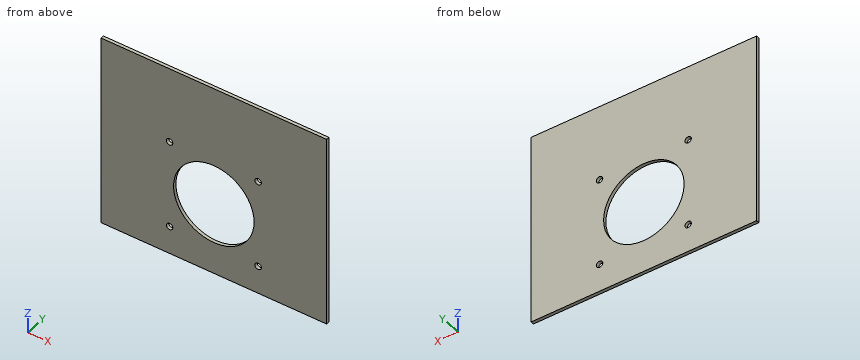
from build123d import *

# Parameters (mm, degrees)
SKETCH_1_W      = 140
SKETCH_1_H      = 120
SKETCH_1_R      = 2
SKETCH_1_R_2    = 25
EXTRUDE_1_DEPTH = 2


with BuildPart() as part:
    # Эскиз1 → Бобышка-Вытянуть1 (new body)
    with BuildSketch(Plane(origin=(0, 0, 0), x_dir=(1, 0, 0), z_dir=(0, 1, 0))):
        with Locations((0, -15)):
            Rectangle(SKETCH_1_W, SKETCH_1_H)
        with Locations((27.5, 27.5)):
            Circle(SKETCH_1_R, mode=Mode.SUBTRACT)
        with Locations((-27.5, 27.5)):
            Circle(SKETCH_1_R, mode=Mode.SUBTRACT)
        with Locations((-27.5, -27.5)):
            Circle(SKETCH_1_R, mode=Mode.SUBTRACT)
        with Locations((27.5, -27.5)):
            Circle(SKETCH_1_R, mode=Mode.SUBTRACT)
        Circle(SKETCH_1_R_2, mode=Mode.SUBTRACT)
    extrude(amount=EXTRUDE_1_DEPTH)


solid = part.part
For this review, take the finished solid that the model builds, in its own axes (mm). Coordinates: 2 decimals unless noted, no trailing zeros. Order: outer loops, then holes, each group sorted by start corner. A loop starts at its lowest first (then second) coordinate and runs counter-clockwise, first axis right, second up. Notation, with made-up numbers: (64, 60.5) -> (88, 60.5) arc R24 cw to (88, 99.5) -> close; hole circle Ø10 at (26.5, 21). An arc over 180 degrees is marked (long way). Return JSON: item names as keys, results as strings.
1. We need section B-B on x = 0. Write out the cut boundary in (y, z).
Answer block:
{"outline": "(0, -45) -> (2, -45) -> (2, -25) -> (0, -25) -> close; (0, 25) -> (2, 25) -> (2, 75) -> (0, 75) -> close"}
2. We need section A-A on z = 27.5. Write out the cut boundary in (x, y).
Answer block:
{"outline": "(-70, 0) -> (-29.5, 0) -> (-29.5, 2) -> (-70, 2) -> close; (-25.5, 0) -> (25.5, 0) -> (25.5, 2) -> (-25.5, 2) -> close; (29.5, 0) -> (70, 0) -> (70, 2) -> (29.5, 2) -> close"}
3. We need section C-C on y = 1.1. Write out the cut boundary in (x, z).
Answer block:
{"outline": "(-70, -45) -> (70, -45) -> (70, 75) -> (-70, 75) -> close; hole circle Ø4 at (-27.5, -27.5); hole circle Ø4 at (-27.5, 27.5); hole circle Ø50 at (0, 0); hole circle Ø4 at (27.5, -27.5); hole circle Ø4 at (27.5, 27.5)"}
4. We need section D-D on z = 0. Write out the cut boundary in (x, y), and give its area (3 significant figures).
Answer block:
{"outline": "(-70, 0) -> (-25, 0) -> (-25, 2) -> (-70, 2) -> close; (25, 0) -> (70, 0) -> (70, 2) -> (25, 2) -> close", "area": "180 mm²"}
5. For line 1 (X direction, y = 1.35, z = -27.5); line 2 (Z direction, x = 27.5, y = 1.15); line 3 (X direction, y = 1.2, z = 0), list the stretches that pass through material, from the lowest coordinate up. Write a range as from..to.
Answer block:
{"line 1": "-70..-29.5, -25.5..25.5, 29.5..70", "line 2": "-45..-29.5, -25.5..25.5, 29.5..75", "line 3": "-70..-25, 25..70"}
